Source: CAD feature listing. Evaluate the final solid. Frame: model axes, mm. Face numbers are marked on the shaded views. A direction names the side the tool comes from. Coordinates: 2 decimals unless noted, no trailing zeros. Write each loop counter-clockwise with the first axis right and the second up, starting at its lowest first coordinate (ties: lowest second). Pieces come first, ordered by that corner, then holes. Notation, with made-up numbers: M -21.75,14.25 L 16.25,14.25 A9 cw 16.25,27.25 Z; hole C 31,-3 d10. An arc over 180 degrees is marked long. Write item = value, one per line. Start each with the question number.
1. Pin query (flat end, axial travel): pin 1 Ø10 at (y, z) = (4, 43) entering from -X; pin 2 Ø1 at (y, z) = (1.5, 31) entering from +X; pin 3 Ø1.5 at (y, z) = (-3.5, 19.5) entering from -X; pin 4 Ø6 at (x, y) = (3.5, -7) entering from -Z. Return the tip coordinate at first contact, or that it passes through.
2. Section query B-B (x = 0). Output: boundary loops of the cut face in (y, z), then the cut area to 3 significant figures.
3. Access query for the marked faces 5 and 6. Directions: +Z, -Z, +X, -X, +Y, -Y. A direction counts if a zero-diameter tool reaches every point of the face in a straight line with its end or side. Return the directions, or none.
4. Section query A-A (z = 13). Output: boundary loops of the cut face in (x, y).
5. Line query: line 1 along X through (y, z) = (7, 4); line 2 along Z through (x, y) = (5.75, 7.25); line 3 along Z through (x, y) = (-4.5, 4.75). Output: solid intervals per line, ascending.
6. Pull-direction query (Y, two-part tool) for the marked faces 1, 2, 3 and 4; classes: pulls with the +Y half, pulls with the -Y half, needs draft (parallel to the pull), parting line crosses it, or undercut.
7. Section query C-C (z = 41). Output: boundary loops of the cut face in (x, y), then the cut area to 3 significant figures.
```python
from build123d import *

# Parameters (mm, degrees)
F0_R     = 11.43
F1_DEPTH = 3.81
F3_DEPTH = 12.7
F4_R     = 4.191
F5_DEPTH = 57.15
F6_DEPTH = 57.15
F7_SIZE  = 1.27
F8_DEPTH = 12.7


with BuildPart() as f1:
    # F0 (on Top) → F1 (new body)
    with BuildSketch(Plane.XY):
        Circle(F0_R)
    extrude(amount=F1_DEPTH)

    # F2 (on face) → F3 (join)
    with BuildSketch(Plane.XY.offset(3.81)):
        with BuildLine():
            ThreePointArc((8.7246484395, -0.8189496979), (8.7534068589, -0.4099236057), (8.763, 0))
            ThreePointArc((8.763, 0), (8.4427240898, 2.3474622346), (7.5053076703, 4.5233312696))
            ThreePointArc((7.5053076703, 4.5233312696), (6.8511892809, 5.4636411337), (6.0800099832, 6.3105980385))
            ThreePointArc((6.0800099832, 6.3105980385), (3.8021232059, 7.8951901894), (1.143, 8.6881367393))
            ThreePointArc((1.143, 8.6881367393), (0, 8.763), (-1.143, 8.6881367393))
            ThreePointArc((-1.143, 8.6881367393), (-3.8021232059, 7.8951901894), (-6.0800099832, 6.3105980385))
            ThreePointArc((-6.0800099832, 6.3105980385), (-6.8511892809, 5.4636411337), (-7.5053076703, 4.5233312696))
            ThreePointArc((-7.5053076703, 4.5233312696), (-8.5432932944, 1.9499509443), (-8.7246484395, -0.8189496979))
            ThreePointArc((-8.7246484395, -0.8189496979), (-8.5432932944, -1.9499509443), (-8.2159655844, -3.0476349052))
            ThreePointArc((-8.2159655844, -3.0476349052), (-6.8511892809, -5.4636411337), (-4.7994486704, -7.3318116083))
            ThreePointArc((-4.7994486704, -7.3318116083), (-3.8021232059, -7.8951901894), (-2.7398338384, -8.323669836))
            ThreePointArc((-2.7398338384, -8.323669836), (0, -8.763), (2.7398338384, -8.323669836))
            ThreePointArc((2.7398338384, -8.323669836), (3.8021232059, -7.8951901894), (4.7994486704, -7.3318116083))
            ThreePointArc((4.7994486704, -7.3318116083), (6.8511892809, -5.4636411337), (8.2159655844, -3.0476349052))
            ThreePointArc((8.2159655844, -3.0476349052), (8.5432932944, -1.9499509443), (8.7246484395, -0.8189496979))
        make_face()
    extrude(amount=F3_DEPTH)

    # F4 (on face) → F5 (join)
    with BuildSketch(Plane.XY.offset(16.51)):
        Circle(F4_R)
    extrude(amount=F5_DEPTH)

    # F4 (on face) → F6 (join)
    with BuildSketch(Plane.XY.offset(16.51)):
        Circle(F4_R)
    extrude(amount=F6_DEPTH)

    # F7
    f7_edges = [f1.edges().sort_by_distance(p)[0] for p in [
        (-11.43, 0, 0),
    ]]
    chamfer(f7_edges, length=F7_SIZE)

    # F2 (on face) → F8 (join)
    with BuildSketch(Plane.XY.offset(3.81)):
        with BuildLine():
            ThreePointArc((8.7246484395, -0.8189496979), (8.7534068589, -0.4099236057), (8.763, 0))
            ThreePointArc((8.763, 0), (8.4427240898, 2.3474622346), (7.5053076703, 4.5233312696))
            ThreePointArc((7.5053076703, 4.5233312696), (6.8511892809, 5.4636411337), (6.0800099832, 6.3105980385))
            ThreePointArc((6.0800099832, 6.3105980385), (3.8021232059, 7.8951901894), (1.143, 8.6881367393))
            ThreePointArc((1.143, 8.6881367393), (0, 8.763), (-1.143, 8.6881367393))
            ThreePointArc((-1.143, 8.6881367393), (-3.8021232059, 7.8951901894), (-6.0800099832, 6.3105980385))
            ThreePointArc((-6.0800099832, 6.3105980385), (-6.8511892809, 5.4636411337), (-7.5053076703, 4.5233312696))
            ThreePointArc((-7.5053076703, 4.5233312696), (-8.5432932944, 1.9499509443), (-8.7246484395, -0.8189496979))
            ThreePointArc((-8.7246484395, -0.8189496979), (-8.5432932944, -1.9499509443), (-8.2159655844, -3.0476349052))
            ThreePointArc((-8.2159655844, -3.0476349052), (-6.8511892809, -5.4636411337), (-4.7994486704, -7.3318116083))
            ThreePointArc((-4.7994486704, -7.3318116083), (-3.8021232059, -7.8951901894), (-2.7398338384, -8.323669836))
            ThreePointArc((-2.7398338384, -8.323669836), (0, -8.763), (2.7398338384, -8.323669836))
            ThreePointArc((2.7398338384, -8.323669836), (3.8021232059, -7.8951901894), (4.7994486704, -7.3318116083))
            ThreePointArc((4.7994486704, -7.3318116083), (6.8511892809, -5.4636411337), (8.2159655844, -3.0476349052))
            ThreePointArc((8.2159655844, -3.0476349052), (8.5432932944, -1.9499509443), (8.7246484395, -0.8189496979))
        make_face()
        with BuildLine():
            ThreePointArc((6.0800099832, 6.3105980385), (6.8511892809, 5.4636411337), (7.5053076703, 4.5233312696))
            Line((7.5053076703, 4.5233312696), (8.7553493037, 5.5202062073))
            Line((8.7553493037, 5.5202062073), (7.3300516166, 7.3074729762))
            Line((7.3300516166, 7.3074729762), (6.0800099832, 6.3105980385))
        make_face()
        with BuildLine():
            Line((10.2834248601, -1.174730244), (8.7246484395, -0.8189496979))
            ThreePointArc((8.7246484395, -0.8189496979), (8.5432932944, -1.9499509443), (8.2159655844, -3.0476349052))
            Line((8.2159655844, -3.0476349052), (9.7747420051, -3.4034154512))
            Line((9.7747420051, -3.4034154512), (10.2834248601, -1.174730244))
        make_face()
        with BuildLine():
            ThreePointArc((-1.143, 8.6881367393), (0, 8.763), (1.143, 8.6881367393))
            Line((1.143, 8.6881367393), (1.143, 10.287))
            Line((1.143, 10.287), (-1.143, 10.287))
            Line((-1.143, 10.287), (-1.143, 8.6881367393))
        make_face()
        with BuildLine():
            Line((5.4931694403, -8.7723376303), (4.7994486704, -7.3318116083))
            ThreePointArc((4.7994486704, -7.3318116083), (3.8021232059, -7.8951901894), (2.7398338384, -8.323669836))
            Line((2.7398338384, -8.323669836), (3.4335546083, -9.7641958579))
            Line((3.4335546083, -9.7641958579), (5.4931694403, -8.7723376303))
        make_face()
        with BuildLine():
            ThreePointArc((-7.5053076703, 4.5233312696), (-6.8511892809, 5.4636411337), (-6.0800099832, 6.3105980385))
            Line((-6.0800099832, 6.3105980385), (-7.3300516166, 7.3074729762))
            Line((-7.3300516166, 7.3074729762), (-8.7553493037, 5.5202062073))
            Line((-8.7553493037, 5.5202062073), (-7.5053076703, 4.5233312696))
        make_face()
        with BuildLine():
            Line((-3.4335546083, -9.7641958579), (-2.7398338384, -8.323669836))
            ThreePointArc((-2.7398338384, -8.323669836), (-3.8021232059, -7.8951901894), (-4.7994486704, -7.3318116083))
            Line((-4.7994486704, -7.3318116083), (-5.4931694403, -8.7723376303))
            Line((-5.4931694403, -8.7723376303), (-3.4335546083, -9.7641958579))
        make_face()
        with BuildLine():
            ThreePointArc((-8.2159655844, -3.0476349052), (-8.5432932944, -1.9499509443), (-8.7246484395, -0.8189496979))
            Line((-8.7246484395, -0.8189496979), (-10.2834248601, -1.174730244))
            Line((-10.2834248601, -1.174730244), (-9.7747420051, -3.4034154512))
            Line((-9.7747420051, -3.4034154512), (-8.2159655844, -3.0476349052))
        make_face()
    extrude(amount=F8_DEPTH)


solid = f1.part
```
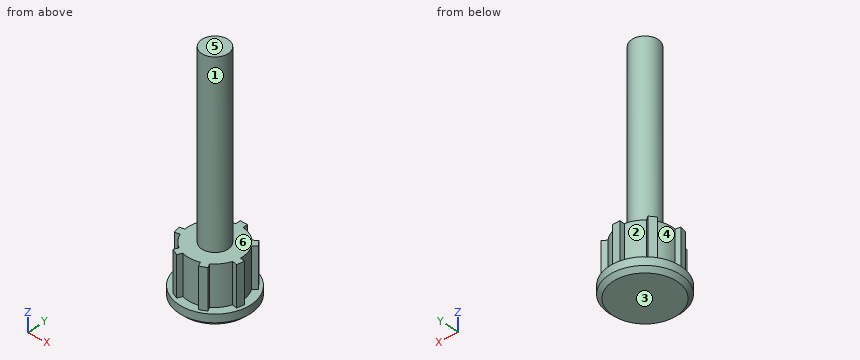
Results are:
q1.pin_1 = -4.19
q1.pin_2 = 4.07
q1.pin_3 = -3.16
q1.pin_4 = 0
q2.outline = M -11.43,1.27 L -10.16,0 L 10.16,0 L 11.43,1.27 L 11.43,3.81 L 10.29,3.81 L 10.29,16.51 L 4.19,16.51 L 4.19,73.66 L -4.19,73.66 L -4.19,16.51 L -8.76,16.51 L -8.76,3.81 L -11.43,3.81 Z
q2.area = 806 mm^2
q3.face_5 = +Z, +X, -X, +Y, -Y
q3.face_6 = +Z
q4.outline = M -10.28,-1.17 L -9.77,-3.4 L -8.22,-3.05 A8.76 ccw -4.8,-7.33 L -5.49,-8.77 L -3.43,-9.76 L -2.74,-8.32 A8.76 ccw 2.74,-8.32 L 3.43,-9.76 L 5.49,-8.77 L 4.8,-7.33 A8.76 ccw 8.22,-3.05 L 9.77,-3.4 L 10.28,-1.17 L 8.72,-0.82 A8.76 ccw 7.51,4.52 L 8.76,5.52 L 7.33,7.31 L 6.08,6.31 A8.76 ccw 1.14,8.69 L 1.14,10.29 L -1.14,10.29 L -1.14,8.69 A8.76 ccw -6.08,6.31 L -7.33,7.31 L -8.76,5.52 L -7.51,4.52 A8.76 ccw -8.72,-0.82 Z
q5.line_1 = -7.58 to -6.94, -5.27 to 5.27, 6.94 to 7.58
q5.line_2 = 0 to 3.81
q5.line_3 = 0 to 16.51
q6.face_1 = parting line crosses it
q6.face_2 = pulls with the +Y half
q6.face_3 = needs draft
q6.face_4 = undercut
q7.outline = C 0,0 d8.38
q7.area = 55.2 mm^2
